Source: CAD feature listing. Evaluate the final solid. Frame: model axes, mm. Give positions to 0.01 mm unless a question says otherwise; leave off trailing zeros. Loops run counter-clockwise (first coordinate to the right, second up) from the corner with the lowest first, then second, coordinate; pieces in that order, holes last. Notation, with made-up numbers: M -31,59.25 L -3,59.25 A22 ccw -3,79.25 Z; hole C -21,11 d1. An arc over 180 degrees is marked long. Put each result on its own line as item: value.
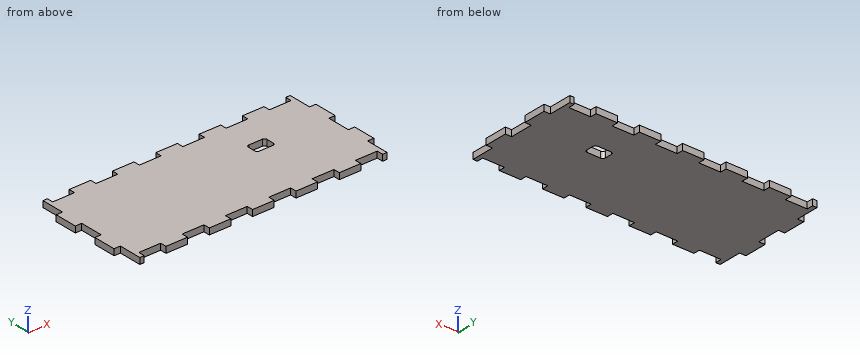
Autodesk Inventor part; units mm, degrees
ref_plane "YZ Plane" through (0, 0, 0) normal (1, 0, 0) x (0, 1, 0)
ref_plane "XZ Plane" through (0, 0, 0) normal (0, 1, 0) x (-1, 0, 0)
ref_plane "XY Plane" through (0, 0, 0) normal (0, 0, 1) x (1, 0, 0)
sketch "Sketch1" plane through (0, 0, 0) normal (0, 0, 1) x (1, 0, 0)
  line L0 (-105, -46) -> (105, -46)
  line L1 (105, -46) -> (105, 46)
  line L2 (105, 46) -> (-105, 46)
  line L3 (-105, 46) -> (-105, -46)
  line L4 (-105, -46) -> (105, 46) construction
  line L5 (105, -46) -> (-105, 46) construction
  point P0 (0, 0)
  dimension "d0" = 210
  dimension "d1" = 92
extrude "Extrusion1" add sketch "Sketch1" along normal blind 5
sketch "Sketch2" plane through (0, 0, 5) normal (0, 0, 1) x (1, 0, 0)
  line L0 (39, 16.1) -> (54, 16.1)
  line L1 (54, 16.1) -> (54, 6.1)
  line L2 (54, 6.1) -> (39, 6.1)
  line L3 (39, 6.1) -> (39, 16.1)
  line L4 (-3, 9.6) -> (85, 9.6) construction
  line L5 (85, 9.6) -> (85, 8) construction
  line L6 (85, 8) -> (-3, 8) construction
  line L7 (-3, 8) -> (-3, 9.6) construction
  line L8 (-105, -46) -> (105, -46) construction
  line L9 (7.25, 15.6) -> (17.25, 15.6)
  line L10 (17.25, 15.6) -> (17.25, 10.6)
  line L11 (17.25, 10.6) -> (7.25, 10.6)
  line L12 (7.25, 10.6) -> (7.25, 15.6)
  line L13 (105, -46) -> (105, 46)
  line L14 (17.25, 10.6) -> (7.25, 15.6) construction
  line L15 (17.25, 15.6) -> (7.25, 10.6) construction
  line L16 (54, 6.1) -> (39, 16.1) construction
  line L17 (39, 6.1) -> (54, 16.1) construction
  point P0 (0, 0)
  point P1 (85, 8.8)
  point P2 (54, 11.1)
  point P3 (12.25, 13.1)
  point P4 (12.25, 13.1)
  point P5 (46.5, 11.1)
  point P6 (46.5, 11.1)
  dimension "d4" = 1.6
  dimension "d5" = 55.6
  dimension "d7" = 15
  dimension "d8" = 10
  dimension "d9" = 10
  dimension "d10" = 5
  dimension "d12" = 88
  dimension "d13" = 20
  dimension "d17" = 3.5
  dimension "d18" = 72.75
  dimension "d19" = 1.5
  dimension "d20" = 38.5
extrude "Extrusion2" cut sketch "Sketch2" against normal blind 5 contours L0 L1 L2 L3
fillet "Fillet1" radius 2 4 edges at (39, 16.1, 2.5) (39, 6.1, 2.5) (54, 6.1, 2.5) (54, 16.1, 2.5)
sketch "Sketch3" plane through (0, 0, 5) normal (0, 0, 1) x (1, 0, 0)
  line L0 (-8.75, 46) -> (-26.35, 46)
  line L1 (-26.35, 46) -> (-26.35, 40.9)
  line L2 (-26.35, 40.9) -> (-8.75, 40.9)
  line L3 (-8.75, 40.9) -> (-8.75, 46)
  line L4 (-43.75, 46) -> (-61.35, 46)
  line L5 (-61.35, 46) -> (-61.35, 40.9)
  line L6 (-61.35, 40.9) -> (-43.75, 40.9)
  line L7 (-43.75, 40.9) -> (-43.75, 46)
  line L8 (-78.75, 46) -> (-96.35, 46)
  line L9 (-96.35, 46) -> (-96.35, 40.9)
  line L10 (-96.35, 40.9) -> (-78.75, 40.9)
  line L11 (-78.75, 40.9) -> (-78.75, 46)
  line L12 (0, 0) -> (0, 46) construction
  line L13 (78.75, 40.9) -> (78.75, 46)
  line L14 (96.35, 40.9) -> (78.75, 40.9)
  line L15 (96.35, 46) -> (96.35, 40.9)
  line L16 (78.75, 46) -> (96.35, 46)
  line L17 (8.75, 40.9) -> (8.75, 46)
  line L18 (26.35, 40.9) -> (8.75, 40.9)
  line L19 (8.75, 46) -> (26.35, 46)
  line L20 (26.35, 46) -> (26.35, 40.9)
  line L21 (43.75, 40.9) -> (43.75, 46)
  line L22 (61.35, 46) -> (61.35, 40.9)
  line L23 (43.75, 46) -> (61.35, 46)
  line L24 (61.35, 40.9) -> (43.75, 40.9)
  line L25 (0, 0) -> (105, 0) construction
  line L26 (-96.35, -40.9) -> (-78.75, -40.9)
  line L27 (-78.75, -40.9) -> (-78.75, -46)
  line L28 (-78.75, -46) -> (-96.35, -46)
  line L29 (-61.35, -40.9) -> (-43.75, -40.9)
  line L30 (-43.75, -40.9) -> (-43.75, -46)
  line L31 (-43.75, -46) -> (-61.35, -46)
  line L32 (-26.35, -46) -> (-26.35, -40.9)
  line L33 (-26.35, -40.9) -> (-8.75, -40.9)
  line L34 (-96.35, -46) -> (-96.35, -40.9)
  line L35 (-61.35, -46) -> (-61.35, -40.9)
  line L36 (-8.75, -40.9) -> (-8.75, -46)
  line L37 (-8.75, -46) -> (-26.35, -46)
  line L38 (8.75, -40.9) -> (8.75, -46)
  line L39 (26.35, -40.9) -> (8.75, -40.9)
  line L40 (8.75, -46) -> (26.35, -46)
  line L41 (26.35, -46) -> (26.35, -40.9)
  line L42 (43.75, -40.9) -> (43.75, -46)
  line L43 (61.35, -46) -> (61.35, -40.9)
  line L44 (43.75, -46) -> (61.35, -46)
  line L45 (61.35, -40.9) -> (43.75, -40.9)
  line L46 (78.75, -40.9) -> (78.75, -46)
  line L47 (78.75, -46) -> (96.35, -46)
  line L48 (96.35, -46) -> (96.35, -40.9)
  line L49 (96.35, -40.9) -> (78.75, -40.9)
  line L50 (105, 46) -> (-105, 46)
  line L51 (-105, 46) -> (-105, -46)
  line L52 (-105, -46) -> (105, -46)
  line L53 (105, -46) -> (105, 46)
  line L54 (-105, 46) -> (-99.9, 46)
  line L55 (-99.9, 46) -> (-99.9, 27.5)
  line L56 (-99.9, 27.5) -> (-105, 27.5)
  line L57 (-105, 27.5) -> (-105, 46)
  line L58 (-105, -46) -> (-99.9, -46)
  line L59 (-99.9, -46) -> (-99.9, -27.5)
  line L60 (-99.9, -27.5) -> (-105, -27.5)
  line L61 (-105, -27.5) -> (-105, -46)
  line L62 (-105, -9.25) -> (-99.9, -9.25)
  line L63 (-99.9, -9.25) -> (-99.9, 9.25)
  line L64 (-99.9, 9.25) -> (-105, 9.25)
  line L65 (-105, 9.25) -> (-105, -9.25)
  line L66 (105, 46) -> (99.9, 46)
  line L67 (99.9, 46) -> (99.9, 27.5)
  line L68 (99.9, 27.5) -> (105, 27.5)
  line L69 (105, 27.5) -> (105, 46)
  line L70 (105, -46) -> (99.9, -46)
  line L71 (99.9, -46) -> (99.9, -27.5)
  line L72 (99.9, -27.5) -> (105, -27.5)
  line L73 (105, -27.5) -> (105, -46)
  line L74 (105, -9.25) -> (99.9, -9.25)
  line L75 (99.9, -9.25) -> (99.9, 9.25)
  line L76 (99.9, 9.25) -> (105, 9.25)
  line L77 (105, 9.25) -> (105, -9.25)
  point P0 (-17.55, 40.9)
  point P1 (-52.55, 40.9)
  point P2 (-87.55, 40.9)
  point P3 (87.55, 40.9)
  point P4 (17.55, 40.9)
  point P5 (52.55, 40.9)
  point P6 (-87.55, -40.9)
  point P7 (-52.55, -40.9)
  point P8 (-17.55, -40.9)
  point P9 (0, -46)
  point P10 (17.55, -40.9)
  point P11 (52.55, -40.9)
  point P12 (87.55, -40.9)
  point P13 (-105, 0)
  dimension "d27" = 17.55
  dimension "d28" = 17.6
  dimension "d29" = 5.1
  dimension "d30" = 35
  dimension "d32" = 210
  dimension "d35" = 92
  dimension "d38" = 18.5
extrude "Extrusion3" cut sketch "Sketch3" against normal blind 5 contours L3 L2 L1 L0 | L19 L20 L18 L17 | L7 L6 L5 L4 | L23 L22 L24 L21 | L11 L10 L9 L8 | L16 L15 L14 L13 | L55 L56 L51 L50 | L50 L53 L68 L67 | L64 L63 L62 L51 | L53 L74 L75 L76 | L60 L59 L52 L51 | L53 L52 L71 L72 | L34 L26 L27 L28 | L47 L46 L49 L48 | L35 L29 L30 L31 | L44 L42 L45 L43 | L32 L33 L36 L37 | L40 L38 L39 L41
equation "\"d30\" = 0.166667 * d32"
properties part number "Backplate" material "MDF Medium Density Fiberboard"
1. Section query A-A (x = -51). Output: boundary loops of the cut face in (y, z), plus the area to 3 significant figures.
Found:
outline: M -40.9,0 L 40.9,0 L 40.9,5 L -40.9,5 Z
area: 409 mm^2
2. Material intervals for line 1 (X direction, y = 9, z = 4.3); line 2 (X direction, y = 13, z = 3.35); line 3 (Y direction, x = 90.5, z = 3.9), sorted ascending. Write a range as from..to.
Found:
line 1: -99.9..39, 54..99.9
line 2: -105..39, 54..105
line 3: -40.9..40.9
3. Contact query for flat-ended pins moving along their axis: P1, Ø1.5, axis at x = -81, z = 3.5, coming from the -Y side; P2, Ø10, axis at x = 20.5, y = -36, coming from the -Z side; P3, Ø1.5, axis at y = -43, z = 3, coming from the +X side; P4, Ø1.5, axis at y = 42.5, z = 3, coming from the -X side. Output: stop coordinate, or through.
Found:
P1: y = -40.9
P2: z = 0
P3: x = 99.9
P4: x = -99.9
4. Section query B-B (y = -32). Output: boundary loops of the cut face in (x, z).
Found:
outline: M -99.9,0 L 99.9,0 L 99.9,5 L -99.9,5 Z
